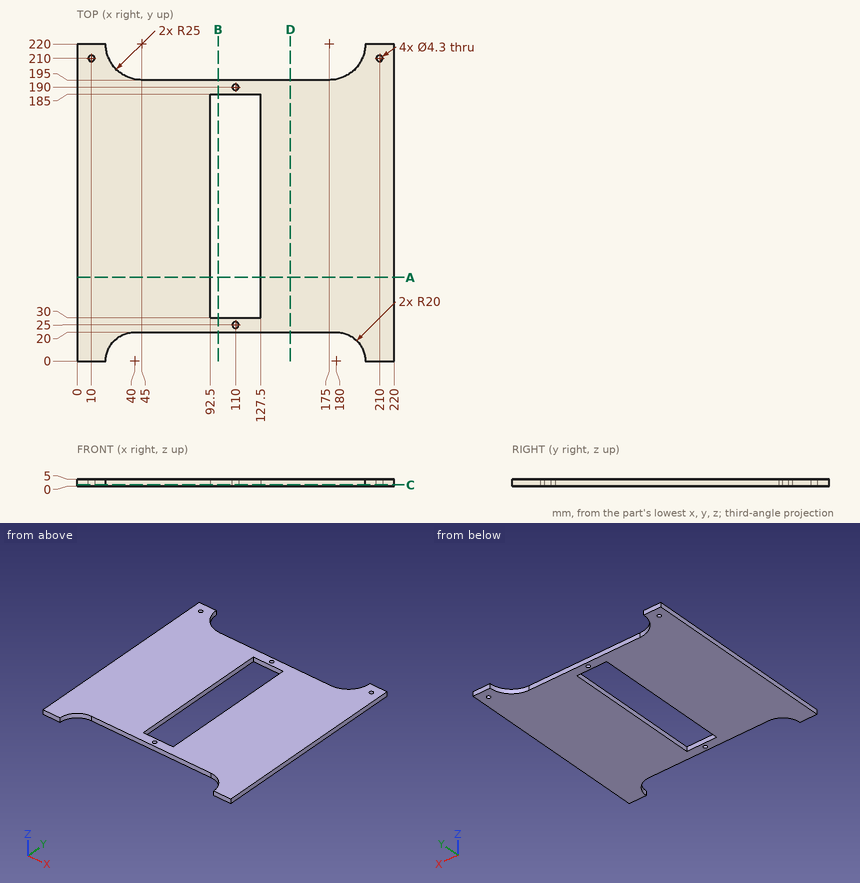
Study the drawing (mm; zero at the part's minimum x, y, z) and answer. Round coordinates to 2 decimals unless told otherwise and drop trailing zeros. Loops run counter-clockwise (first coordinate to the right, second up) from the corner with the lowest first, then second, coordinate; pieces in that order, holes last. Notation, with made-up numbers: M -5,77 L 4,77 A23 cw 4,89 Z; hole C 33,-1.5 d8. An arc over 180 degrees is marked long. One line per question, with ' | ' between items.
Q1. Find section D-D, the plane x = 148. Give the vertices of the cut face in (y, z).
Conclusion:
outline: M 20,0 L 195,0 L 195,5 L 20,5 Z
Q2. Find section B-B, the plane x = 98. Give the vertices of the cut face in (y, z), then the cut area to 3 significant figures.
Conclusion:
outline: M 20,0 L 30,0 L 30,5 L 20,5 Z; M 185,0 L 195,0 L 195,5 L 185,5 Z | area: 100 mm2
Q3. Each of these flat-tipped pins is pushed along its axis until it touches: pin 1 Ø2 at (x, z) = (95, 4.5) entering from -Y; pin 2 Ø5 at (x, y) = (110, 190) entering from +Z; pin 3 Ø2.5 at (x, y) = (210, 210) entering from +Z. Where does it stop, or does it pass through?
Conclusion:
pin 1: stops at y = 20 | pin 2: stops at z = 5 | pin 3: passes through
Q4. Find section C-C, the plane z = 0.85. Give the vertices of the cut face in (x, y), then the cut area to 3 significant figures.
Conclusion:
outline: M 0,0 L 20,0 A20 cw 40,20 L 180,20 A20 cw 200,0 L 220,0 L 220,220 L 200,220 A25 cw 175,195 L 45,195 A25 cw 20,220 L 0,220 Z; hole C 10,210 d4.3; hole M 92.5,30 L 127.5,30 L 127.5,185 L 92.5,185 Z; hole C 110,25 d4.3; hole C 110,190 d4.3; hole C 210,210 d4.3 | area: 35,300 mm2
Q5. Consider line 1 along Y through (x, z) = (110, 3.1); line 2 along Y through (x, z) = (117, 0.3); line 3 along X through (y, z) = (103.5, 2.6). Determine where each line is inside the solid, lowest interval first. Write a range as from..to.
Conclusion:
line 1: y = 20..22.85, 27.15..30, 185..187.85, 192.15..195 | line 2: y = 20..30, 185..195 | line 3: x = 0..92.5, 127.5..220
Q6. Find section A-A, the plane y = 58. Give the vertices of the cut face in (x, z), then the cut area to 3 significant figures.
Conclusion:
outline: M 0,0 L 92.5,0 L 92.5,5 L 0,5 Z; M 127.5,0 L 220,0 L 220,5 L 127.5,5 Z | area: 925 mm2
